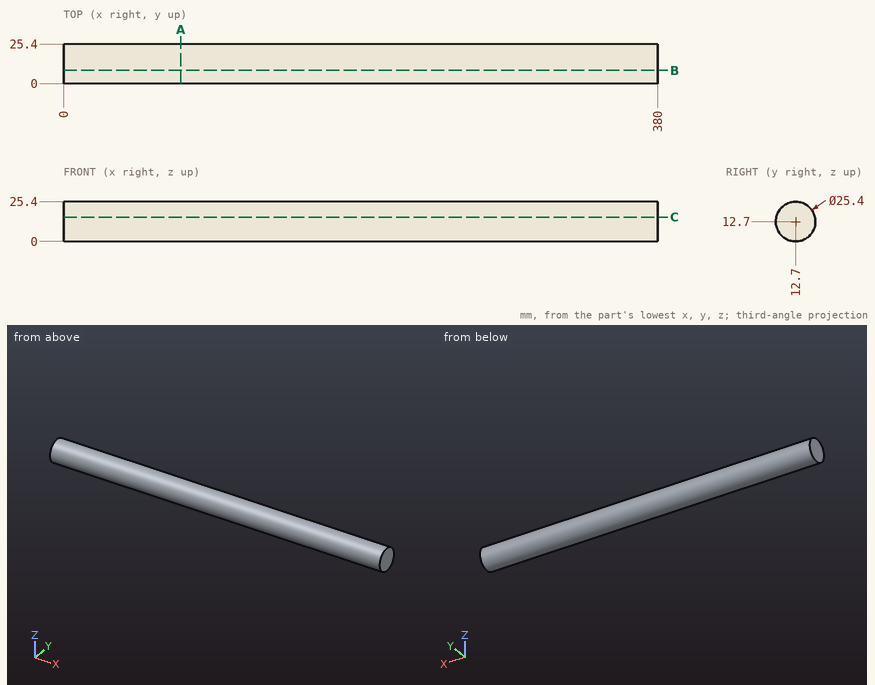
Print and shaded views of the part. All mm, measured from the part's lowest x, y and z. Give positions to 0.01 mm unless a question says otherwise; leave off trailing zeros. Loops run counter-clockwise (first coordinate to the right, second up) from the corner with the lowest first, then second, coordinate; pieces in that order, holes last. Notation, with made-up numbers: (10.25, -8) - (37.25, -8) arc R25 cw to (37.25, 26) - close; hole circle Ø10 at (77.25, 35). An arc over 180 degrees is marked (long way). Use a Markdown table: item, result.
(1) Band-saw the part on A-A (x = 75). Give the cut face in (y, z).
Taken from the geometry:
| item | result |
|---|---|
| outline | circle Ø25.4 at (12.7, 12.7) |
(2) Wall check: line 1 along Y through (x, z) = (65.5, 12); line 2 along Z through (x, y) = (117.5, 13.5); line 3 along Z through (x, y) = (124, 11.5). Give the ranges that are in metal, low to high.
Taken from the geometry:
| item | result |
|---|---|
| line 1 | 0.02 to 25.38 |
| line 2 | 0.03 to 25.37 |
| line 3 | 0.06 to 25.34 |
(3) Drop flat-ended pins along their axis: pin 1 Ø10 at (x, z) = (182.5, 6) entering from -Y; pin 2 Ø1.5 at (x, z) = (309.5, 4.5) entering from -Y; pin 3 Ø1 at (x, z) = (264.5, 17.5) entering from -Y. Give the stop position or say it passes through.
Taken from the geometry:
| item | result |
|---|---|
| pin 1 | y = 0.11 |
| pin 2 | y = 2.41 |
| pin 3 | y = 0.75 |
(4) Band-saw the part on B-B (y = 8.5). Give the cut face in (x, z).
Taken from the geometry:
| item | result |
|---|---|
| outline | (0, 0.71) - (380, 0.71) - (380, 24.69) - (0, 24.69) - close |
(5) Band-saw the part on C-C (z = 15.5). Give the cut face in (x, y), and give its area (3 significant figures).
Taken from the geometry:
| item | result |
|---|---|
| outline | (0, 0.31) - (380, 0.31) - (380, 25.09) - (0, 25.09) - close |
| area | 9,410 mm2 |
